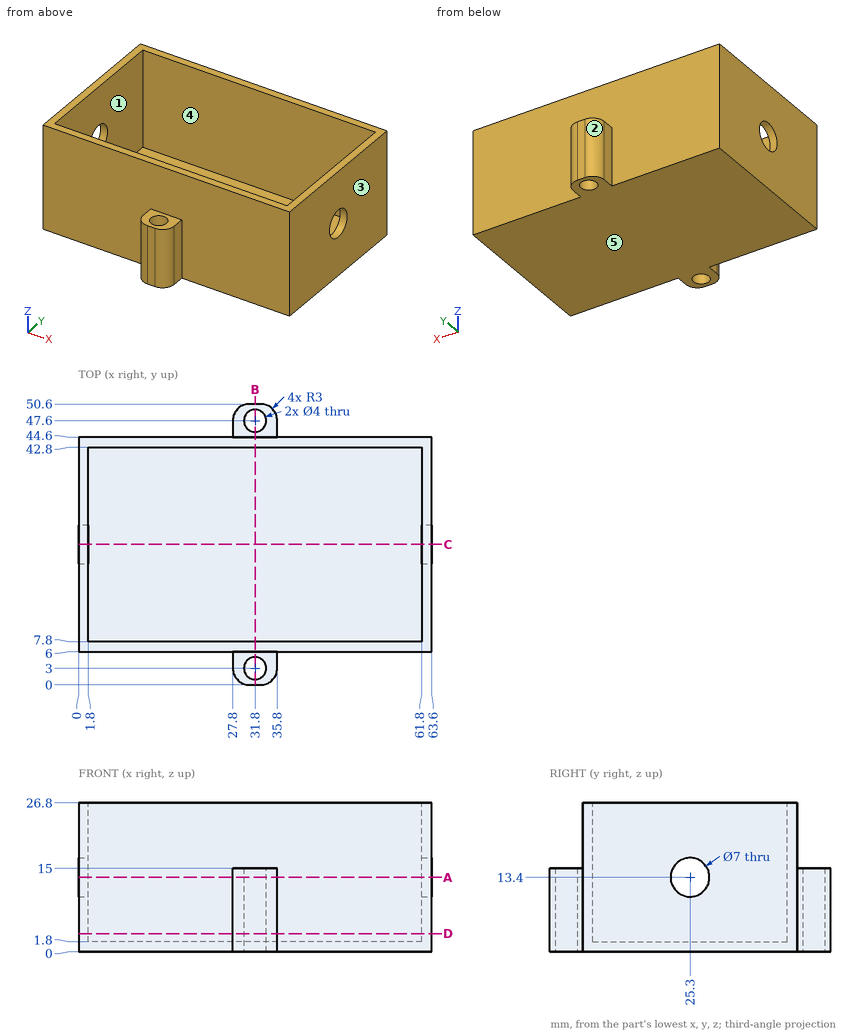
Job drawing, mm, ordinate dimensions from the low corner. One solid piece. A direction names the side the tool comes from. Round coordinates to 2 decimals unless told otherwise and drop trailing zeros. Write each loop counter-clockwise with the first axis right and the second up, starting at its lowest first coordinate (ties: lowest second). Pieces come first, ordered by that corner, then holes.
1) Drill centre lines: probe 1 along Y at (x, z) = (31.8, 11.5); probe 2 along Y at (x, z) = (28.5, 24.75); probe 3 along X at (y, z) = (30, 2.5). Where is each one in solid material? Low to high.
2) Band-saw the part on D-D, the plane z = 3.25. List the corners of the cut face in (x, y).
3) 3-axis set-ups, long thin cutter, end or side, ignore diameter. For the marked faces 4 and 5: which of +Z, -Z, +X, -X, +Y, -Y reach the whole face in a straight line?
4) Band-saw the part on A-A, the plane z = 13.4. Give the number of separate pieces and of enclosed holes in the cut face, and give its area (3 significant figures).
5) Mould opens along X. For the marked faces 1, 2 and 3 say: +X half, -X half, draft (parallel to the pull), parting line (faces both ways), or undercut.
6) Pin check, flat tips, straight feed: pin 1 (1.5 mm diameter, centred on y = 4, z = 8.5, fed in from +X); pin 2 (7.5 mm diameter, centred on x = 17.5, z = 16, fed in from +Y); pin 3 (7.5 mm diameter, centred on x = 45.5, z = 10, fed in from -Y); pin 4 (6.5 mm diameter, centred on y = 25.3, z = 13.4, fed in from +X). Stop position of each tip, or through.
7) Band-saw the part on C-C, the plane y = 25.3. List the corners of the cut face in (x, z), and give its area (3 significant figures).
8) Band-saw the part on B-B, the plane x = 31.8. List the corners of the cut face in (y, z).
Ans:
1. probe 1: y = 0 to 1, 5 to 7.8, 42.8 to 45.6, 49.6 to 50.6
1. probe 2: y = 6 to 7.8, 42.8 to 44.6
1. probe 3: x = 0 to 1.8, 61.8 to 63.6
2. outline: (0, 6) - (27.8, 6) - (27.8, 3) arc R3 ccw to (30.8, 0) - (32.8, 0) arc R3 ccw to (35.8, 3) - (35.8, 6) - (63.6, 6) - (63.6, 44.6) - (35.8, 44.6) - (35.8, 47.6) arc R3 ccw to (32.8, 50.6) - (30.8, 50.6) arc R3 ccw to (27.8, 47.6) - (27.8, 44.6) - (0, 44.6) - close; hole (1.8, 7.8) - (61.8, 7.8) - (61.8, 42.8) - (1.8, 42.8) - close; hole circle Ø4 at (31.8, 3); hole circle Ø4 at (31.8, 47.6)
3. face 4: +Z
3. face 5: -Z, +X, -X, +Y, -Y
4. separate pieces: 2
4. enclosed holes: 2
4. area: 393 mm2
5. face 1: undercut
5. face 2: -X half
5. face 3: +X half
6. pin 1: stops at x = 35.8
6. pin 2: stops at y = 44.6
6. pin 3: stops at y = 6
6. pin 4: passes through
7. outline: (0, 0) - (63.6, 0) - (63.6, 9.9) - (61.8, 9.9) - (61.8, 1.8) - (1.8, 1.8) - (1.8, 9.9) - (0, 9.9) - close; (0, 16.9) - (1.8, 16.9) - (1.8, 26.8) - (0, 26.8) - close; (61.8, 16.9) - (63.6, 16.9) - (63.6, 26.8) - (61.8, 26.8) - close
7. area: 179 mm2
8. outline: (0, 0) - (1, 0) - (1, 15) - (0, 15) - close; (5, 0) - (45.6, 0) - (45.6, 15) - (44.6, 15) - (44.6, 26.8) - (42.8, 26.8) - (42.8, 1.8) - (7.8, 1.8) - (7.8, 26.8) - (6, 26.8) - (6, 15) - (5, 15) - close; (49.6, 0) - (50.6, 0) - (50.6, 15) - (49.6, 15) - close
